The listing builds one solid part. Answer for the finished solid, in the listing's coordinates (mm). A direction names the side the tool comes from. Coordinates: 2 decimals unless noted, no trailing zeros. Order: outer loops, then holes, each group sorted by start corner. A loop starts at its lowest first (then second) coordinate and runs counter-clockwise, first axis right, second up. Notation, with made-up numbers: (75, 41) -> (90, 41) arc R32 cw to (90, 74) -> close; hole circle Ø8 at (56, 6.25). An arc over 180 degrees is marked (long way). Return JSON: item names as keys, results as strings.
from build123d import *

# Parameters (mm, degrees)
F0_W     = 70
F0_H     = 50
F0_W_2   = 60
F0_H_2   = 40
F1_DEPTH = 12.5
F2_R     = 2.5
F3_DEPTH = 50.001


with BuildPart() as f1:
    # F0 (on Top) → F1 (new body, symmetric)
    with BuildSketch(Plane.XY):
        Rectangle(F0_W, F0_H)
        Rectangle(F0_W_2, F0_H_2, mode=Mode.SUBTRACT)
    extrude(amount=F1_DEPTH, both=True)

    # F2 (on face) → F3 (cut, through all)
    with BuildSketch(Plane.XZ.offset(25)):
        with Locations((-24, 0)):
            Circle(F2_R)
        Circle(F2_R)
        with Locations((24, 0)):
            Circle(F2_R)
    extrude(amount=-F3_DEPTH, mode=Mode.SUBTRACT)


solid = f1.part
1. This flat-tipped pin is pushed along its axis until it touches: pin 1 Ø4 at (x, z) = (24, 0) entering from -Y. Where does it stop, or does it pass through?
Answer block:
{"pin 1": "passes through"}
2. The part is cut by section D-D on x = 0. Give the vertices of the cut face in (y, z), and give its area (3 significant figures).
Answer block:
{"outline": "(-25, -12.5) -> (-20, -12.5) -> (-20, -2.5) -> (-25, -2.5) -> close; (-25, 2.5) -> (-20, 2.5) -> (-20, 12.5) -> (-25, 12.5) -> close; (20, -12.5) -> (25, -12.5) -> (25, -2.5) -> (20, -2.5) -> close; (20, 2.5) -> (25, 2.5) -> (25, 12.5) -> (20, 12.5) -> close", "area": "200 mm2"}
3. Determine the mould class of faces 3 (the face through (21.5, -22.5, 0.1)), 4 (the face through (0, -22, 12.5)), 5 (the face through (0, 25, 3)) for opening direction Z: pulls with the +Z half, pulls with the -Z half, needs draft (parallel to the pull), parting line crosses it, or undercut.
Answer block:
{"face 3": "undercut", "face 4": "pulls with the +Z half", "face 5": "needs draft"}
4. The part is cut by section A-A on x = 13. Give the vertices of the cut face in (y, z).
Answer block:
{"outline": "(-25, -12.5) -> (-20, -12.5) -> (-20, 12.5) -> (-25, 12.5) -> close; (20, -12.5) -> (25, -12.5) -> (25, 12.5) -> (20, 12.5) -> close"}
5. Consider line 1 (Y direction, x = 1.5, z = -7.25); line 2 (X direction, y = -3, z = -11); line 3 (Z direction, x = 24, y = -22). Determine where each line is inside the solid, lowest interval first. Write a range as from..to.
Answer block:
{"line 1": "y = -25..-20, 20..25", "line 2": "x = -35..-30, 30..35", "line 3": "z = -12.5..-2.5, 2.5..12.5"}
6. For faces 1 (the face through (0, -22, -12.5)), 2 (the face through (30, 0, 0)), determine the directions among +Z, -Z, +X, -X, +Y, -Y from which every point of the face is accessible in a straight line to the end or side of a thin tool.
Answer block:
{"face 1": "-Z, +X, -X, +Y, -Y", "face 2": "+Z, -Z"}
7. The part is cut by section B-B on y = -0.5. Give the vertices of the cut face in (x, z).
Answer block:
{"outline": "(-35, -12.5) -> (-30, -12.5) -> (-30, 12.5) -> (-35, 12.5) -> close; (30, -12.5) -> (35, -12.5) -> (35, 12.5) -> (30, 12.5) -> close"}
8. The part is cut by section C-C on z = 0. Give the number of separate pieces and of enclosed holes in the cut face, and give its area (3 significant figures).
Answer block:
{"separate pieces": "6", "enclosed holes": "0", "area": "950 mm2"}
